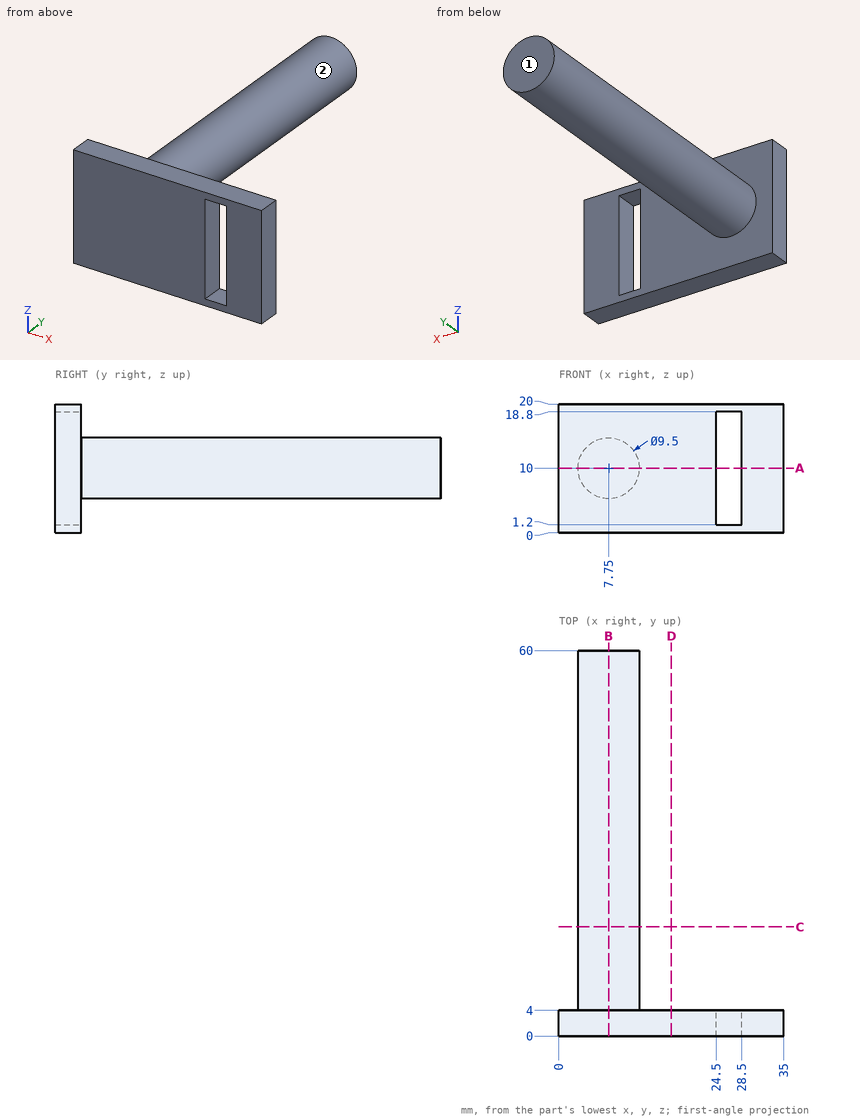
Answer from the drawing. Dimensions are ordinates in mm from the lowest x, y and z of the part. A direction names the side the tool comes from. Coordinates: 2 decimals unless noted, no trailing zeros. Order: outer loops, then holes, each group sorted by start corner. A loop starts at its lowest first (then second) coordinate and runs counter-clockwise, first axis right, second up. Notation, with made-up numbers: (54, 40.25) - (95, 40.25) arc R18 cw to (95, 46.25) - close; hole circle Ø11 at (-31.75, -38). An arc over 180 degrees is marked (long way). Use one line per item in the form item = value.
(1) Straight lines are drawn through the part: L1, parallel to Y at x = 14, z = 17.25; L2, parallel to X at y = 53, z = 13.5; L3, parallel to X at y = 47, z = 9.75. For each, find the intervals that lie inside material, in ascending order.
Computed values:
L1 = 0 to 4
L2 = 4.54 to 10.96
L3 = 3.01 to 12.49
(2) Section D-D, the plane x = 17.5 is taken. Give the vertices of the cut face in (y, z), then the cut area to 3 significant figures.
Computed values:
outline = (0, 0) - (4, 0) - (4, 20) - (0, 20) - close
area = 80.0 mm²
(3) Which of the six approach directions +Z, -Z, +X, -X, +Y, -Y give full straight-line access (tool end or side, diameter ignored) to the marked faces 1 and 2?
Computed values:
face_1 = +Z, -Z, +X, -X, +Y
face_2 = +Y
(4) Section A-A, the plane z = 10 is taken. Give the vertices of the cut face in (x, y).
Computed values:
outline = (0, 0) - (24.5, 0) - (24.5, 4) - (12.5, 4) - (12.5, 60) - (3, 60) - (3, 4) - (0, 4) - close; (28.5, 0) - (35, 0) - (35, 4) - (28.5, 4) - close
(5) Given pin 1 Ø2 at (x, y) = (8, 37.5) entering from +Z; pin 2 Ø10 at (x, z) = (22.5, 10.5) entering from +Y; pin 3 Ø8 at (y, z) = (28.5, 7) entering from +X, each flat-ended and moving along its own axis, determine where each tip first touches the part or whether it passes through.
Computed values:
pin_1 = 14.75
pin_2 = 4
pin_3 = 12.5
(6) Section B-B, the plane x = 7.75 is taken. Give the vertices of the cut face in (y, z), then the cut area to 3 significant figures.
Computed values:
outline = (0, 0) - (4, 0) - (4, 5.25) - (60, 5.25) - (60, 14.75) - (4, 14.75) - (4, 20) - (0, 20) - close
area = 612 mm²
(7) Section C-C, the plane y = 17 is taken. Give the vertices of the cut face in (x, z), then the cut area to 3 significant figures.
Computed values:
outline = circle Ø9.5 at (7.75, 10)
area = 70.9 mm²
